```python
from build123d import *

# Parameters (mm, degrees)
SKETCH1_W               = 60
SKETCH1_H               = 72
BOSS_EXTRUDE1_DEPTH     = 6
SKETCH2_W               = 10
SKETCH2_H               = 6
CUT_EXTRUDE1_DEPTH      = 1
CUT_EXTRUDE1_DEPTH_BACK = 7
SKETCH3_R               = 1.5
CUT_EXTRUDE2_DEPTH      = 1
CUT_EXTRUDE2_DEPTH_BACK = 7
SKETCH6_W               = 6
SKETCH6_H               = 66
BOSS_EXTRUDE2_DEPTH     = 27.5
SKETCH7_W               = 6
SKETCH7_H               = 66
BOSS_EXTRUDE3_DEPTH     = 7.5
SKETCH8_R               = 1.5
CUT_EXTRUDE3_DEPTH      = 7


with BuildPart() as part:
    # Sketch1 → Boss-Extrude1 (new body)
    with BuildSketch(Plane.XY):
        Rectangle(SKETCH1_W, SKETCH1_H)
    extrude(amount=BOSS_EXTRUDE1_DEPTH)

    # Sketch2 → Cut-Extrude1 (cut, two sides)
    with BuildSketch(Plane.XY.offset(6)) as cut_extrude1_sk:
        with Locations((-25, 33)):
            Rectangle(SKETCH2_W, SKETCH2_H)
        with Locations((-25, -33)):
            Rectangle(SKETCH2_W, SKETCH2_H)
        with Locations((25, -33)):
            Rectangle(SKETCH2_W, SKETCH2_H)
        with Locations((25, 33)):
            Rectangle(SKETCH2_W, SKETCH2_H)
    extrude(amount=CUT_EXTRUDE1_DEPTH, mode=Mode.SUBTRACT)
    extrude(cut_extrude1_sk.sketch, amount=-CUT_EXTRUDE1_DEPTH_BACK, mode=Mode.SUBTRACT)

    # Sketch3 → Cut-Extrude2 (cut, two sides)
    with BuildSketch(Plane.XY.offset(6)) as cut_extrude2_sk:
        with Locations((-15, 12)):
            Circle(SKETCH3_R)
        with Locations((-15, -12)):
            Circle(SKETCH3_R)
        with Locations((15, -12)):
            Circle(SKETCH3_R)
        with Locations((15, 12)):
            Circle(SKETCH3_R)
    extrude(amount=CUT_EXTRUDE2_DEPTH, mode=Mode.SUBTRACT)
    extrude(cut_extrude2_sk.sketch, amount=-CUT_EXTRUDE2_DEPTH_BACK, mode=Mode.SUBTRACT)

    # Sketch6 → Boss-Extrude2 (add)
    with BuildSketch(Plane(origin=(30, 0, 0), x_dir=(0, 0, -1), z_dir=(1, 0, 0))):
        with Locations((-3, 0)):
            Rectangle(SKETCH6_W, SKETCH6_H)
    extrude(amount=BOSS_EXTRUDE2_DEPTH)

    # Sketch7 → Boss-Extrude3 (add)
    with BuildSketch(Plane.ZY.offset(30)):
        with Locations((3, 0)):
            Rectangle(SKETCH7_W, SKETCH7_H)
    extrude(amount=BOSS_EXTRUDE3_DEPTH)

    # Sketch8 → Cut-Extrude3 (cut, through all)
    with BuildSketch(Plane.XY.offset(6)):
        with Locations((54, -29)):
            Circle(SKETCH8_R)
        with Locations((54, 29)):
            Circle(SKETCH8_R)
        with Locations((-34, 29)):
            Circle(SKETCH8_R)
        with Locations((-34, -29)):
            Circle(SKETCH8_R)
    extrude(amount=-CUT_EXTRUDE3_DEPTH, mode=Mode.SUBTRACT)


solid = part.part
```
Here's how the part is built. I have some questions about the finished solid (model axes, mm). A direction names the side the tool comes from. Give positions to 0.01 mm unless a question says otherwise; leave off trailing zeros. Write each loop counter-clockwise with the first axis right and the second up, starting at its lowest first coordinate (ties: lowest second). Pieces come first, ordered by that corner, then holes. Notation, with made-up numbers: (76, 35.25) -> (115, 35.25) arc R28 ccw to (115, 61.25) -> close; hole circle Ø5 at (48.25, 0.25). An arc over 180 degrees is marked (long way). Write each question's results on one line, items separated by ' | '.
Item 1: We'd pull the mould along X, two halves only. Please class faces 6 (the face through (0, -36, 3)), 7 (the face through (-37.5, 0, 3)), 8 (the face through (-35.11, 30.01, 3.04)): pulls with the +X half, pulls with the -X half, needs draft (parallel to the pull), parting line crosses it, or undercut.
Output:
face 6: needs draft | face 7: pulls with the -X half | face 8: undercut
Item 2: If I drill on L1, parallel to Y at x = 15, z = 2.85; L2, parallel to Y at x = -34, z = 3.1; L3, parallel to X at y = 31.5, z = 5.1, over which ranges is the centre line in solid material (lowest first)?
Output:
L1: y = -36 to -13.5, -10.5 to 10.5, 13.5 to 36 | L2: y = -33 to -30.5, -27.5 to 27.5, 30.5 to 33 | L3: x = -37.5 to -30, -20 to 20, 30 to 57.5
Item 3: For pin 1 Ø1.5 at (x, z) = (21, 3) entering from -Y; pin 2 Ø1.8 at (x, y) = (54, 29) entering from -Z; pin 3 Ø1.8 at (x, z) = (42, 3.5) entering from -Y; pin 4 Ø1.8 at (x, z) = (-24.5, 4) entering from +Y, each with a flat end and sliding along its axis, tell me the tip position at first contact or that it passes through.
Output:
pin 1: stops at y = -30 | pin 2: passes through | pin 3: stops at y = -33 | pin 4: stops at y = 30
Item 4: On a 3-axis mill with a long thin cutter (end or side, diameter ignored), from which of +Z, -Z, +X, -X, +Y, -Y can I reach the whole of each face in a straight line? I mean faces 1 (the face through (11, -1, 6)), 2 (the face through (25, 30, 3)), 3 (the face through (-34, 33, 3)), 4 (the face through (-25, -30, 3)), 5 (the face through (-34, -33, 3)). Say none if no direction works.
Output:
face 1: +Z, +X, -X, +Y, -Y | face 2: +Z, -Z, +Y | face 3: +Z, -Z, -X, +Y | face 4: +Z, -Z, -Y | face 5: +Z, -Z, -X, -Y
Item 5: Suppose I cut it at B-B on y = 12. Write out the boundary of the cut face in (x, z).
Output:
outline: (-37.5, 0) -> (-16.5, 0) -> (-16.5, 6) -> (-37.5, 6) -> close; (-13.5, 0) -> (13.5, 0) -> (13.5, 6) -> (-13.5, 6) -> close; (16.5, 0) -> (57.5, 0) -> (57.5, 6) -> (16.5, 6) -> close
Item 6: Suppose I cut it at D-D on x = 49. Write out the boundary of the cut face in (y, z).
Output:
outline: (-33, 0) -> (33, 0) -> (33, 6) -> (-33, 6) -> close
Item 7: Suppose I cut it at A-A on x = 15. Write out the boundary of the cut face in (y, z).
Output:
outline: (-36, 0) -> (-13.5, 0) -> (-13.5, 6) -> (-36, 6) -> close; (-10.5, 0) -> (10.5, 0) -> (10.5, 6) -> (-10.5, 6) -> close; (13.5, 0) -> (36, 0) -> (36, 6) -> (13.5, 6) -> close
Item 8: Suppose I cut it at C-C on z = 1.05. Give the number of separate pieces and of enclosed holes in the cut face, plus the area to 3 significant figures.
Output:
separate pieces: 1 | enclosed holes: 8 | area: 6,330 mm^2
